Geometry check sheet. Reference: the model listing, model coordinates, mm. Coordinates: 2 decimals unless noted, no trailing zeros. Order: outer loops, then holes, each group sorted by start corner. A loop starts at its lowest first (then second) coordinate and runs counter-clockwise, first axis right, second up. Notation, with made-up numbers: M -4.5,5.25 L 14.5,5.25 A28 ccw 14.5,27.25 Z; hole C 17,-12 d3. An arc over 180 degrees is marked long. Use CSV: the item, a comma, the result in double quotes. Start each with the question number.
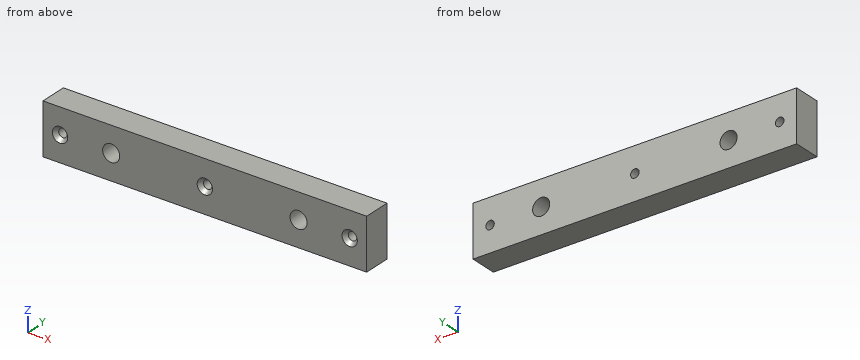
```python
from build123d import *

# Parameters (mm, degrees)
F0_W           = 190
F0_H           = 30
F1_DEPTH       = 16
F3_D           = 5
F3_CSINK_D     = 9
F3_CSINK_ANGLE = 82
F4_D           = 10
F6_D           = 10


with BuildPart() as f1:
    # F0 (on Front) → F1 (new body)
    with BuildSketch(Plane.XZ):
        with Locations((95, -15)):
            Rectangle(F0_W, F0_H)
    extrude(amount=F1_DEPTH)

    # F3 (through all)
    with Locations(Plane.XZ.offset(16)):
        with Locations((10, -15), (95, -15), (180, -15), (180, -15)):
            CounterSinkHole(F3_D / 2, F3_CSINK_D / 2, counter_sink_angle=F3_CSINK_ANGLE)

    # F4 (through all)
    with Locations(Plane.XZ.offset(16)):
        with Locations((40, -15), (156, -52.788887)):
            Hole(F4_D / 2)

    # F6 (through all)
    with Locations(Plane.XZ.offset(16)):
        with Locations((150, -15)):
            Hole(F6_D / 2)


solid = f1.part
```
1) Section check B-B on y = -8. Record the boundary of the cut face in (x, z).
2) Section check A-A on x = 40. Record the boundary of the cut face in (y, z), then the cut area to 3 significant figures.
3) Gauge pin test, flat end, axial feed: P1, Ø4.5, axis at x = 10, z = -15, coming from the -Y side. Record the tip position at first contact, or that the pin passes through.
4) Section check C-C on z = -15. State how many separate pieces and enclosed holes the cut face has, then the cut area to 3 significant figures.
5) Material ranges on line 1 along Z through (x, y) = (10, -9.75); line 2 along Z through (x, y) = (40, -11.25); line 3 along X through (y, z) = (-5.25, -17), recorded low to high.
6) Section check D-D on x = 10. Record the boundary of the cut face in (y, z).
Results are:
1,outline,"M 0,-30 L 190,-30 L 190,0 L 0,0 Z; hole C 10,-15 d5; hole C 40,-15 d10; hole C 95,-15 d5; hole C 150,-15 d10; hole C 180,-15 d5"
2,outline,"M -16,-30 L 0,-30 L 0,-20 L -16,-20 Z; M -16,-10 L 0,-10 L 0,0 L -16,0 Z"
2,area,"320 mm²"
3,P1,"passes through"
4,separate pieces,"6"
4,enclosed holes,"0"
4,area,"2,470 mm²"
5,line 1,"z = -30 to -17.5, -12.5 to 0"
5,line 2,"z = -30 to -20, -10 to 0"
5,line 3,"x = 0 to 8.5, 11.5 to 35.42, 44.58 to 93.5, 96.5 to 145.42, 154.58 to 178.5, 181.5 to 190"
6,outline,"M -16,-30 L 0,-30 L 0,-17.5 L -13.7,-17.5 L -16,-19.5 Z; M -16,-10.5 L -13.7,-12.5 L 0,-12.5 L 0,0 L -16,0 Z"
